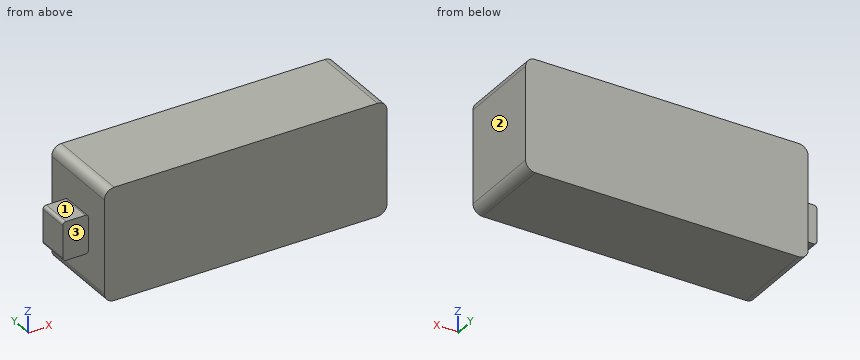
```python
from build123d import *

# Parameters (mm, degrees)
CELL_PACK_DEPTH = 26.5
CONNECTOR_START = 8
CONNECTOR_DEPTH = 10


with BuildPart() as part:
    # SK_1 → Cell_Pack (new body)
    with BuildSketch(Plane(origin=(0, 0, 0), x_dir=(1, 0, 0), z_dir=(0, 1, 0))):
        with BuildLine():
            Line((-41, -17.5), (41, -17.5))
            ThreePointArc((41, -17.5), (43.121320344, -16.621320344), (44, -14.5))
            Line((44, -14.5), (44, 14.5))
            ThreePointArc((44, 14.5), (43.121320344, 16.621320344), (41, 17.5))
            Line((41, 17.5), (-41, 17.5))
            ThreePointArc((-41, 17.5), (-43.121320344, 16.621320344), (-44, 14.5))
            Line((-44, 14.5), (-44, -14.5))
            ThreePointArc((-44, -14.5), (-43.121320344, -16.621320344), (-41, -17.5))
        make_face()
    extrude(amount=CELL_PACK_DEPTH)

    # SK_2 → Connector (add)
    with BuildSketch(Plane(origin=(0, 0, 0), x_dir=(1, 0, 0), z_dir=(0, 1, 0)).offset(CONNECTOR_START)):
        with BuildLine():
            Line((-51, -6), (-45, -6))
            ThreePointArc((-45, -6), (-44.292893219, -5.707106781), (-44, -5))
            Line((-44, -5), (-44, 5))
            ThreePointArc((-44, 5), (-44.292893219, 5.707106781), (-45, 6))
            Line((-45, 6), (-51, 6))
            ThreePointArc((-51, 6), (-51.707106781, 5.707106781), (-52, 5))
            Line((-52, 5), (-52, -5))
            ThreePointArc((-52, -5), (-51.707106781, -5.707106781), (-51, -6))
        make_face()
    extrude(amount=CONNECTOR_DEPTH)


solid = part.part
```
Source: CAD feature listing. Evaluate the final solid. Frame: model axes, mm. Face numbers are marked on the shaded views. A direction names the side the tool comes from. Coordinates: 2 decimals unless noted, no trailing zeros. Write each loop counter-clockwise with the first axis right and the second up, starting at its lowest first coordinate (ties: lowest second). Pieces come first, ordered by that corner, then holes. Notation, with made-up numbers: (-14, 25) - (-6, 25) arc R16 cw to (-6, 31) - close; hole circle Ø1 at (69, 61.5). An arc over 180 degrees is marked (long way). Answer as a JSON object with one key per item and string values.
Q1. Material intervals for line 1 (X direction, y = 22.5, z = -11.5); line 2 (Z direction, x = -45, y = 15); line 3 (X direction, y = 21.75, z = 16.5), sorted ascending. Write a range as [from, to].
Ans:
{"line 1": "x = [-44, 44]", "line 2": "z = [-6, 6]", "line 3": "x = [-43.24, 43.24]"}
Q2. Section query A-A, the plane y = 22. Output: boundary loops of the cut face in (x, z).
Ans:
{"outline": "(-44, -14.5) arc R3 ccw to (-41, -17.5) - (41, -17.5) arc R3 ccw to (44, -14.5) - (44, 14.5) arc R3 ccw to (41, 17.5) - (-41, 17.5) arc R3 ccw to (-44, 14.5) - close"}
Q3. First-contact query: pin 1 Ø2 at (y, z) = (19.5, -10) entering from -X; pin 2 Ø4 at (x, z) = (-46.5, -2) entering from +Y; pin 3 Ø2.5 at (x, z) = (-48.5, 2.5) entering from -Y. Flat tips, straight axial feed; report the tip coordinate or a pass-through.
Ans:
{"pin 1": "stops at x = -44", "pin 2": "stops at y = 18", "pin 3": "stops at y = 8"}
Q4. Set-up query: the marked faces 1, 2 and 3. Return all of +Z, -Z, +X, -X, +Y, -Y with unobstructed straight access to the full face (end or side cutting, diameter ignored); none if empty.
Ans:
{"face 1": "+Z, -X, +Y, -Y", "face 2": "+Z, -Z, +X, +Y, -Y", "face 3": "+Z, -Z, -X, -Y"}
Q5. Section query B-B, the plane z = -13. Output: boundary loops of the cut face in (x, y), plus the area to 3 significant figures.
Ans:
{"outline": "(-44, 0) - (44, 0) - (44, 26.5) - (-44, 26.5) - close", "area": "2,330 mm2"}
